```python
from build123d import *

# Parameters (mm, degrees)
BOSS_EXTRU_2_START      = 8
ESQUISSE4_R             = 1
BOSS_EXTRU_2_DEPTH      = 8
ENL_V_MAT_EXTRU_1_DEPTH = 20.178438414
ENL_V_MAT_EXTRU_2_REACH = 21.178
ESQUISSE6_W             = 2
ESQUISSE6_H             = 5.5
CONG_1_R                = 0.25
ESQUISSE7_W             = 1
ESQUISSE7_H             = 4.690983006
ENL_V_MAT_EXTRU_3_DEPTH = 0.2
CONG_2_R                = 0.25
CONG_2_OF_SYM_TRIE1_R   = 0.25


with BuildPart() as part:
    # Esquisse1 → Révolution1 (revolve)
    with BuildSketch(Plane.XY, mode=Mode.PRIVATE) as r_volution1_sk:
        with BuildLine():
            Line((2, 9), (2, 17))
            Line((2, 17), (0.45, 17))
            Line((0.45, 17), (0.45, 12))
            Line((0.45, 12), (1, 12))
            Line((1, 12), (1, 0))
            Line((1, 0), (4.5, 0))
            ThreePointArc((4.5, 0), (4.676776695, 0.073223305), (4.75, 0.25))
            Line((4.75, 0.25), (4.75, 11.75))
            ThreePointArc((4.75, 11.75), (4.676776695, 11.926776695), (4.5, 12))
            Line((4.5, 12), (3.75, 12))
            Line((3.75, 12), (3.75, 11))
            Line((3.75, 11), (4.25, 11))
            Line((4.25, 11), (4.25, 9))
            Line((4.25, 9), (2, 9))
        make_face()
    revolve(r_volution1_sk.sketch.rotate(Axis((0, 0, 0), (0, 1, 0)), 90), axis=Axis((0, 0, 0), (0, 1, 0)))

    # Esquisse4 → Boss.-Extru.2 (add)
    with BuildSketch(Plane.XZ.offset(BOSS_EXTRU_2_START)):
        with BuildLine():
            Line((-2.5, -2.75), (2.5, -2.75))
            ThreePointArc((2.5, -2.75), (2.676776695, -2.676776695), (2.75, -2.5))
            Line((2.75, -2.5), (2.75, 2.5))
            ThreePointArc((2.75, 2.5), (2.676776695, 2.676776695), (2.5, 2.75))
            Line((2.5, 2.75), (-2.5, 2.75))
            ThreePointArc((-2.5, 2.75), (-2.676776695, 2.676776695), (-2.75, 2.5))
            Line((-2.75, 2.5), (-2.75, -2.5))
            ThreePointArc((-2.75, -2.5), (-2.676776695, -2.676776695), (-2.5, -2.75))
        make_face()
        with Locations(Location((0, 0, 0), (0, 0, 270))):
            Circle(ESQUISSE4_R, mode=Mode.SUBTRACT)
    extrude(amount=-BOSS_EXTRU_2_DEPTH)

    # Esquisse5 → Enlèv. mat.-Extru.1 (cut, through all)
    with BuildSketch(Plane(origin=(2.75, 0, 0), x_dir=(0, 0, -1), z_dir=(1, 0, 0))):
        with BuildLine():
            Line((-2.5, -8), (0, -8))
            ThreePointArc((0, -8), (-1.48525742, -7.564413618), (-2.5, -6.395643924))
            Line((-2.5, -6.395643924), (-2.5, -8))
        make_face()
        with BuildLine():
            Line((2.5, -8), (2.5, -6.395643924))
            ThreePointArc((2.5, -6.395643924), (1.48525742, -7.564413618), (0, -8))
            Line((0, -8), (2.5, -8))
        make_face()
        with BuildLine():
            Line((-2.75, -8), (-2.5, -8))
            Line((-2.5, -8), (-2.5, -6.395643924))
            ThreePointArc((-2.5, -6.395643924), (-2.686773158, -5.83630197), (-2.75, -5.25))
            Line((-2.75, -5.25), (-2.75, -8))
        make_face()
        with BuildLine():
            Line((2.75, -8), (2.75, -5.25))
            ThreePointArc((2.75, -5.25), (2.686773158, -5.83630197), (2.5, -6.395643924))
            Line((2.5, -6.395643924), (2.5, -8))
            Line((2.5, -8), (2.75, -8))
        make_face()
        with BuildLine():
            ThreePointArc((-0.75, -5.25), (0, -6), (0.75, -5.25))
            Line((0.75, -5.25), (-0.75, -5.25))
        make_face()
        with BuildLine():
            Line((-0.75, -5.25), (0.75, -5.25))
            ThreePointArc((0.75, -5.25), (0, -4.5), (-0.75, -5.25))
        make_face()
    extrude(amount=-ENL_V_MAT_EXTRU_1_DEPTH, mode=Mode.SUBTRACT)

    # Esquisse6 → Enlèv. mat.-Extru.2 (cut, up to next)
    with BuildSketch(Plane.XY.offset(-2.75), mode=Mode.PRIVATE) as enl_v_mat_extru_2_sk1:
        with Locations((0, -5.25)):
            Rectangle(ESQUISSE6_W, ESQUISSE6_H)
    enl_v_mat_extru_2_tool1 = extrude(enl_v_mat_extru_2_sk1.sketch, amount=ENL_V_MAT_EXTRU_2_REACH, mode=Mode.PRIVATE) & part.part
    add(enl_v_mat_extru_2_tool1.solids().sort_by_distance((0, -5.25, -2.75))[0], mode=Mode.SUBTRACT)

    # Congé1
    cong_1_edges = [part.edges().sort_by_distance(p)[0] for p in [
        (1, -7.194543649, -1.944543647),
        (-1, -7.194543648, -1.944543648),
        (-1, -3.875, -2.75),
        (0, -2.5, -2.75),
        (1, -3.875, -2.75),
        (0, -7.811737691, 1),
    ]]
    fillet(cong_1_edges, radius=CONG_1_R)

    # Esquisse7 → Enlèv. mat.-Extru.3 (cut)
    with BuildSketch(Plane.ZY.offset(2.75)):
        with Locations((0, -2.345491503)):
            Rectangle(ESQUISSE7_W, ESQUISSE7_H)
    enl_v_mat_extru_3 = extrude(amount=-ENL_V_MAT_EXTRU_3_DEPTH, mode=Mode.SUBTRACT)

    # Congé2
    # the kernel refuses this fillet: 0.25 mm, written as the material it adds along each edge
    with BuildSketch(Plane(origin=(-2.55, -5.303355441, 0.5), x_dir=(-1.0, 0, -1.569855356819468e-12), z_dir=(0, 1, 0))) as cong_2_piece_1_section:
        with BuildLine():
            CenterArc((0.25, -0.244948974), CONG_2_R, 101.536959033, 78.463040967)
            Line((0, -0.244948974), (-0.005, -0.244948974))
            Line((-0.005, -0.244948974), (-0.005, 0))
            Line((-0.005, 0), (0, 0.005))
            ThreePointArc((0, 0.005), (0.1, 0.005), (0.199, 0.004898979))
            Line((0.199, 0.004898979), (0.2, 0))
        make_face()
    cong_2_piece_1 = extrude(amount=5.915727877, mode=Mode.PRIVATE)
    cong_2_piece_1 = cong_2_piece_1 - Plane(origin=(-2.600107301, -5.25, 0), x_dir=(0, 0, 1), z_dir=(1, 0, 0)) * Cylinder(0.75, 13, mode=Mode.PRIVATE)
    add(cong_2_piece_1)
    with BuildSketch(Plane(origin=(-2.55, 0.612372436, -0.5), x_dir=(-1.0, 0, 1.569855356819468e-12), z_dir=(0, -1, 0))) as cong_2_piece_2_section:
        with BuildLine():
            CenterArc((0.25, -0.244948974), CONG_2_R, 101.536959033, 78.463040967)
            Line((0, -0.244948974), (-0.005, -0.244948974))
            Line((-0.005, -0.244948974), (-0.005, 0))
            Line((-0.005, 0), (0, 0.005))
            ThreePointArc((0, 0.005), (0.1, 0.005), (0.199, 0.004898979))
            Line((0.199, 0.004898979), (0.2, 0))
        make_face()
    cong_2_piece_2 = extrude(amount=5.915727877, mode=Mode.PRIVATE)
    cong_2_piece_2 = cong_2_piece_2 - Plane(origin=(-2.599890025, -5.25, 0), x_dir=(0, 0, 1), z_dir=(1, 0, 0)) * Cylinder(0.75, 13, mode=Mode.PRIVATE)
    add(cong_2_piece_2)

    # Symétrie1: Enlèv. mat.-Extru.3 across plane
    add(enl_v_mat_extru_3.mirror(Plane(origin=(0, 0, 0), x_dir=(0, 0, 1), z_dir=(1, 0, 0))), mode=Mode.SUBTRACT)

    # Congé2 of Symétrie1
    # the kernel refuses this fillet: 0.25 mm, written as the material it adds along each edge
    with BuildSketch(Plane(origin=(2.55, -5.303355441, 0.5), x_dir=(0, 0, -1), z_dir=(0, 1, 0))) as cong_2_of_sym_trie1_piece_1_section:
        with BuildLine():
            CenterArc((0.244948974, -0.25), CONG_2_OF_SYM_TRIE1_R, 90, 78.463040967)
            Line((0, -0.2), (-0.004898979, -0.199))
            ThreePointArc((-0.004898979, -0.199), (-0.005, -0.1), (-0.005, 0))
            Line((-0.005, 0), (0, 0.005))
            Line((0, 0.005), (0.244948974, 0.005))
            Line((0.244948974, 0.005), (0.244948974, 0))
        make_face()
    cong_2_of_sym_trie1_piece_1 = extrude(amount=5.915727877, mode=Mode.PRIVATE)
    cong_2_of_sym_trie1_piece_1 = cong_2_of_sym_trie1_piece_1 - Plane(origin=(2.600107302, -5.25, 0), x_dir=(0, 0, 1), z_dir=(1, 0, 0)) * Cylinder(0.75, 13, mode=Mode.PRIVATE)
    add(cong_2_of_sym_trie1_piece_1)
    with BuildSketch(Plane(origin=(2.55, 0.612372436, -0.5), x_dir=(1.0, 0, 1.569855356819468e-12), z_dir=(0, -1, 0))) as cong_2_of_sym_trie1_piece_2_section:
        with BuildLine():
            CenterArc((0.25, 0.244948974), CONG_2_OF_SYM_TRIE1_R, 180, 78.463040967)
            Line((0, 0.244948974), (-0.005, 0.244948974))
            Line((-0.005, 0.244948974), (-0.005, 0))
            Line((-0.005, 0), (0, -0.005))
            ThreePointArc((0, -0.005), (0.1, -0.005), (0.199, -0.004898979))
            Line((0.199, -0.004898979), (0.2, 0))
        make_face()
    cong_2_of_sym_trie1_piece_2 = extrude(amount=5.915727877, mode=Mode.PRIVATE)
    cong_2_of_sym_trie1_piece_2 = cong_2_of_sym_trie1_piece_2 - Plane(origin=(2.599890025, -5.25, 0), x_dir=(0, 0, 1), z_dir=(1, 0, 0)) * Cylinder(0.75, 13, mode=Mode.PRIVATE)
    add(cong_2_of_sym_trie1_piece_2)


solid = part.part
```
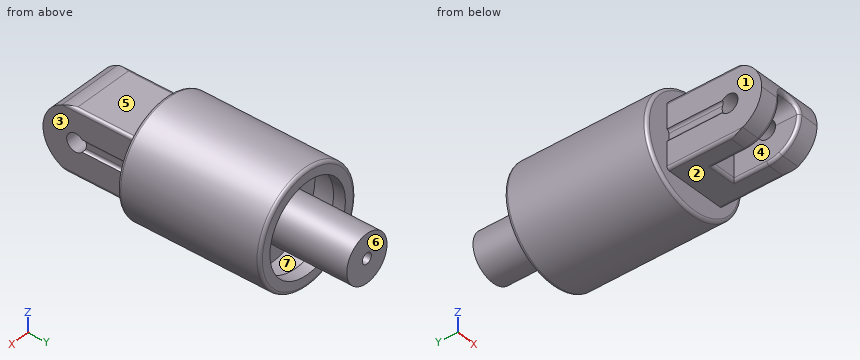
CAD build for the part. Positions are in the model's coordinates, mm. Face numbers are marked on the shaded views. A direction names the side the tool comes from. Coordinates: 2 decimals unless noted, no trailing zeros. Write each loop counter-clockwise with the first axis right and the second up, starting at its lowest first coordinate (ties: lowest second). Pieces come first, ordered by that corner, then holes. Notation, with made-up numbers: (22.5, 70.25) -> (56.5, 70.25) arc R21 cw to (56.5, 84.25) -> close; hole circle Ø2 at (-9.5, 83). An arc over 180 degrees is marked (long way). Use CSV: the item, a comma, the result in double quotes. Start each with the question number.
Item 1: Band-saw the part on B-B, the plane y = 3.75. Write the cut outline in (x, z).
Item 2: Tool access for the marked faces 1, 2, 3 and 4: list every direction of +Z, -Z, +X, -X, +Y, -Y with a clear straight run to the whole face (end or side of a thin tool).
Item 3: Drop flat-ended pins along their axis: P1, Ø2, axis at y = -5, z = -3, coming from the +X side; P2, Ø2, axis at x = -1.5, y = 0, coming from the -Z side; P3, Ø1.5, axis at y = -2.5, z = 0.5, coming from the -X side. Give the stop position or say it passes through.
Item 4: Two-plate mould, pull along Y, no slides. Class the marked faces 5, 6 and 7: +Y half, -Y half, draft (parallel to the pull), parting line (faces both ways), or undercut.
Item 5: Band-saw the part on A-A, the plane y = -1.75. Write the cut outline in (x, z).
Item 6: Wall check: probe 1 along X at (y, z) = (11.75, 0); probe 2 along X at (y, z) = (-2.75, 0.75); probe 3 along Y at (x, z) = (3, 2.75). Give the ranges that are in metal, low to high.
Response values:
1,outline,"circle Ø9.5 at (0, 0); hole circle Ø2 at (0, 0)"
2,face 1,"+Z, -Z, -X, -Y"
2,face 2,"-Z, +X, -X, -Y"
2,face 3,"+Z, -Z, +X, -Y"
2,face 4,"-Z, -Y"
3,P1,"stops at x = 2.75"
3,P2,"stops at z = -4.72"
3,P3,"stops at x = -2.75"
4,face 5,"draft"
4,face 6,"+Y half"
4,face 7,"undercut"
5,outline,"(-2.75, -2.5) arc R0.25 ccw to (-2.5, -2.75) -> (2.5, -2.75) arc R0.25 ccw to (2.75, -2.5) -> (2.75, -0.5) arc R0.25 cw to (2.55, -0.26) -> (2.55, 0.26) arc R0.25 cw to (2.75, 0.5) -> (2.75, 2.5) arc R0.25 ccw to (2.5, 2.75) -> (-2.5, 2.75) arc R0.25 ccw to (-2.75, 2.5) -> (-2.75, 0.5) arc R0.25 cw to (-2.55, 0.26) -> (-2.55, -0.26) arc R0.25 cw to (-2.75, -0.5) -> close; hole circle Ø2 at (0, 0)"
6,probe 1,"x = -4.75 to -3.75, -2 to -1, 1 to 2, 3.75 to 4.75"
6,probe 2,"x = -2.75 to -0.66, 0.66 to 2.75"
6,probe 3,"y = 0 to 9, 11 to 12"
